For this review, take the finished solid that the model builds, in its own axes (mm). Coordinates: 2 decimals unless noted, no trailing zeros. Order: outer loops, then holes, each group sorted by start corner. A loop starts at its lowest first (then second) coordinate and runs counter-clockwise, first axis right, second up.
from build123d import *

# Parameters (mm, degrees)
F1_DEPTH = 5.588
F0_R     = 1.5875
F2_DEPTH = 3.175


with BuildPart() as f1:
    # F0 (on Top) → F1 (new body)
    with BuildSketch(Plane.XY):
        with BuildLine():
            ThreePointArc((-2.799588, 28.616356), (-12.598289, -11.49637), (24.694917, 6.231072))
            ThreePointArc((24.694917, 6.231072), (19.562358, 20.664277), (6.469421, 28.616356))
            ThreePointArc((6.469421, 28.616356), (1.834917, 29.091072), (-2.799588, 28.616356))
        make_face()
        with BuildLine():
            ThreePointArc((-5.369862, -14.225706), (-11.397518, -10.952969), (-16.101802, -5.961661))
            ThreePointArc((-16.101802, -5.961661), (-16.153461, -5.251027), (-16.274676, -4.548904))
            ThreePointArc((-16.274676, -4.548904), (-14.617901, -2.300976), (-12.707877, -0.263846))
            ThreePointArc((-12.707877, -0.263846), (-9.80272, -1.945343), (-6.675045, -3.163954))
            ThreePointArc((-6.675045, -3.163954), (-5.100362, -7.640459), (-2.253338, -11.436929))
            ThreePointArc((-2.253338, -11.436929), (-3.721621, -12.931872), (-5.369862, -14.225706))
        make_face(mode=Mode.SUBTRACT)
        with BuildLine():
            ThreePointArc((-18.082916, -2.351967), (-19.844564, 5.607587), (-18.543271, 13.655228))
            Line((-18.543271, 13.655228), (-17.270199, 14.533076))
            ThreePointArc((-17.270199, 14.533076), (-15.785824, 11.462826), (-13.704401, 8.76144))
            ThreePointArc((-13.704401, 8.76144), (-13.996186, 4.919357), (-13.704401, 1.077274))
            ThreePointArc((-13.704401, 1.077274), (-15.513504, -0.802895), (-17.065671, -2.900195))
            ThreePointArc((-17.065671, -2.900195), (-17.546558, -2.574616), (-18.082916, -2.351967))
        make_face(mode=Mode.SUBTRACT)
        with BuildLine():
            ThreePointArc((22.149822, -1.364534), (17.251466, -9.024046), (9.64394, -14.002755))
            ThreePointArc((9.64394, -14.002755), (9.244871, -12.732225), (8.723306, -11.50688))
            ThreePointArc((8.723306, -11.50688), (11.917547, -7.623779), (14.162866, -3.124869))
            ThreePointArc((14.162866, -3.124869), (17.057838, -2.357953), (19.630023, -0.824041))
            ThreePointArc((19.630023, -0.824041), (20.882224, -1.13018), (22.149822, -1.364534))
        make_face(mode=Mode.SUBTRACT)
        with BuildLine():
            ThreePointArc((-0.539564, -10.602418), (-3.361813, -6.969483), (-4.954739, -2.653711))
            Line((-4.954739, -2.653711), (-0.53185, 3.376688))
            ThreePointArc((-0.53185, 3.376688), (4.442387, 2.774831), (9.417674, 3.36794))
            Line((9.417674, 3.36794), (12.491665, -2.036115))
            ThreePointArc((12.491665, -2.036115), (10.283672, -6.735963), (6.817503, -10.602418))
            ThreePointArc((6.817503, -10.602418), (3.138969, -10.796056), (-0.539564, -10.602418))
        make_face(mode=Mode.SUBTRACT)
        with BuildLine():
            ThreePointArc((20.173145, 0.418834), (20.847319, 4.204631), (20.781009, 8.049416))
            ThreePointArc((20.781009, 8.049416), (21.749844, 10.743143), (22.246701, 13.562352))
            ThreePointArc((22.246701, 13.562352), (23.516492, 6.776863), (22.589715, -0.06392))
            ThreePointArc((22.589715, -0.06392), (21.370847, 0.124476), (20.173145, 0.418834))
        make_face(mode=Mode.SUBTRACT)
        with BuildLine():
            ThreePointArc((-15.963672, 16.307464), (-14.733515, 18.843029), (-13.14645, 21.171891))
            ThreePointArc((-13.14645, 21.171891), (-8.670762, 23.594902), (-3.63687, 24.345036))
            ThreePointArc((-3.63687, 24.345036), (-2.297105, 22.543175), (-1.13104, 20.62433))
            ThreePointArc((-1.13104, 20.62433), (-3.970215, 16.553071), (-5.971208, 12.010815))
            ThreePointArc((-5.971208, 12.010815), (-9.49366, 11.485055), (-12.815938, 10.20187))
            ThreePointArc((-12.815938, 10.20187), (-14.794346, 13.046106), (-15.963672, 16.307464))
        make_face(mode=Mode.SUBTRACT)
        with BuildLine():
            ThreePointArc((1.375797, 27.914656), (-1.246765, 26.971986), (-3.638193, 25.541065))
            ThreePointArc((-3.638193, 25.541065), (-6.82851, 25.352013), (-9.900401, 24.470341))
            ThreePointArc((-9.900401, 24.470341), (-4.500847, 26.973461), (1.375797, 27.914656))
        make_face(mode=Mode.SUBTRACT)
        with BuildLine():
            Line((-0.814806, 4.867908), (-4.685726, 11.308071))
            ThreePointArc((-4.685726, 11.308071), (-2.843515, 15.954202), (0.081828, 20.006689))
            ThreePointArc((0.081828, 20.006689), (4.298062, 20.138545), (8.50931, 19.894825))
            ThreePointArc((8.50931, 19.894825), (11.480397, 16.077327), (13.477047, 11.671189))
            ThreePointArc((13.477047, 11.671189), (11.741579, 8.160706), (9.621952, 4.867908))
            ThreePointArc((9.621952, 4.867908), (4.403573, 4.235942), (-0.814806, 4.867908))
        make_face(mode=Mode.SUBTRACT)
        with BuildLine():
            ThreePointArc((10.484066, 24.194032), (13.488074, 23.481635), (16.356681, 22.340291))
            ThreePointArc((16.356681, 22.340291), (18.980093, 19.513824), (21.061465, 16.267427))
            ThreePointArc((21.061465, 16.267427), (20.915004, 12.905343), (20.173145, 9.622858))
            ThreePointArc((20.173145, 9.622858), (17.24992, 11.144383), (14.049745, 11.931256))
            ThreePointArc((14.049745, 11.931256), (12.086703, 16.392472), (9.114349, 20.255255))
            ThreePointArc((9.114349, 20.255255), (10.099355, 22.120266), (10.484066, 24.194032))
        make_face(mode=Mode.SUBTRACT)
        with BuildLine():
            ThreePointArc((12.790839, 24.948881), (11.385585, 25.277937), (9.95159, 25.441265))
            ThreePointArc((9.95159, 25.441265), (8.440252, 26.514134), (6.784581, 27.347166))
            ThreePointArc((6.784581, 27.347166), (9.877607, 26.37316), (12.790839, 24.948881))
        make_face(mode=Mode.SUBTRACT)
    extrude(amount=F1_DEPTH)

    # F0 (on Top) → F2 (join)
    with BuildSketch(Plane.XY):
        with BuildLine():
            ThreePointArc((-2.799588, 28.616356), (1.834917, 29.091072), (6.469421, 28.616356))
            ThreePointArc((6.469421, 28.616356), (1.834917, 33.749825), (-2.799588, 28.616356))
        make_face()
        with Locations((1.834917, 31.558864)):
            Circle(F0_R, mode=Mode.SUBTRACT)
    extrude(amount=F2_DEPTH)


solid = f1.part
1. Take a section at C-C, the plane x = 15. Give the boundary of the cut face in (y, z), plus the area to 3 significant figures.
Answer below:
outline: (-12.46, 0) - (-11, 0) - (-11, 5.59) - (-12.46, 5.59) - close; (-2.99, 0) - (11.78, 0) - (11.78, 5.59) - (-2.99, 5.59) - close; (22.94, 0) - (24.92, 0) - (24.92, 5.59) - (22.94, 5.59) - close
area: 102 mm2
2. Clearance check with flat-ended pins moving along their axes: pin 1 Ø1 at (y, z) = (-2.5, 4) entering from -X; pin 2 Ø1 at (y, z) = (13.5, 3.5) entering from +X; pin 3 Ø3 at (y, z) = (21.5, 2.5) entering from +X. State where each tip first meets the part, or that it passes through.
Answer below:
pin 1: stops at x = -19.49
pin 2: stops at x = 23.67
pin 3: stops at x = 20.08
3. To check wall thickness, follow L1, parallel to Y at x = -8, z = 1.35; L2, parallel to X at y = 7, z = 2.1; L3, parallel to Y at x = 14.5, z = 1.8. State the ranges of each line that lie inside material, in increasing order.
Answer below:
L1: y = -14.41 to -13.1, -2.71 to 11.81, 23.8 to 25.1, 25.56 to 26.87
L2: x = -21.01 to -19.84, -13.91 to -2.1, 11.05 to 20.87, 23.51 to 24.68
L3: y = -12.8 to -11.38, -3.08 to 11.87, 23.13 to 25.26
4. The part is to be moulded in two halves that separate along Y. For faces 1 (the face through (1.9, 29.09, 4.36)), 2 (the face through (1.5, 3.3, 0)), 3 (the face through (9.84, 26.39, 2.75)), say which applies: +Y half, -Y half, draft (parallel to the pull), parting line (faces both ways), or undercut.
Answer below:
face 1: +Y half
face 2: draft
face 3: undercut
5. Take a section at A-A, the plane y = -4. Give the boundary of the cut face in (x, z), plus the area to 3 significant figures.
Answer below:
outline: (-18.61, 0) - (-15.91, 0) - (-15.91, 5.59) - (-18.61, 5.59) - close; (-6.49, 0) - (-4.62, 0) - (-4.62, 5.59) - (-6.49, 5.59) - close; (11.77, 0) - (13.82, 0) - (13.82, 5.59) - (11.77, 5.59) - close; (20.96, 0) - (22.28, 0) - (22.28, 5.59) - (20.96, 5.59) - close
area: 44.4 mm2
6. Take a section at B-B, the plane x = -7.5. Give the boundary of the cut face in (y, z), plus the area to 3 significant figures.
Answer below:
outline: (-14.64, 0) - (-13.35, 0) - (-13.35, 5.59) - (-14.64, 5.59) - close; (-2.9, 0) - (11.88, 0) - (11.88, 5.59) - (-2.9, 5.59) - close; (23.93, 0) - (25.22, 0) - (25.22, 5.59) - (23.93, 5.59) - close; (25.81, 0) - (27.1, 0) - (27.1, 5.59) - (25.81, 5.59) - close
area: 104 mm2
7. Take a section at D-D, the plane z = 4.2. Give the number of separate pieces and of enclosed holes in the cut face, plus the area to 3 significant figures.
Answer below:
separate pieces: 1
enclosed holes: 10
area: 713 mm2
